For this review, take the finished solid that the model builds, in its own axes (mm). Face numbers are marked on the shaded views. A direction names the side the tool comes from. Round coordinates to 2 decimals unless told otherwise and drop trailing zeros. Order: outer loops, then holes, each group sorted by start corner. A loop starts at its lowest first (then second) coordinate and runs counter-clockwise, first axis right, second up. Notation, with made-up numbers: (8, -6) - (31, -6) arc R12 ccw to (31, 14) - close; hole circle Ø10 at (87, -4). An arc over 180 degrees is marked (long way). Write each question's results on one line, items separated by ' | '. Start each with the question number.
(1) Take a section at B-B, the plane z = -31.5. Give the number of separate pieces and of enclosed holes in the cut face, plus the area to 3 significant figures.
(2) Insertion check: pin 1 Ø4.5 at (x, z) = (35, -10) entering from +Y; pin 2 Ø6.5 at (x, z) = (35, -30) entering from +Y; pin 3 Ø4 at (x, z) = (8, -21) entering from -Y; pin 4 Ø10.5 at (x, z) = (37, -20.5) entering from -Y. Each pin has a flat end and moves straight along its axis. Give the tip position at first contact, or say it passes through.
(3) For the marked faces 5 and 6, list the 3-axis set-ups (+Z, -Z, +X, -X, +Y, -Y) from which the entire face can be reached by the end or side of a thin tool; tool diameter is ignored.
(4) For L1, parallel to Z at x = 35, y = 12; L2, parallel to X at y = 9.75, z = -30; L3, parallel to Z at x = 14.5, y = 7.75, list the stretches that pass through material, from the lowest coordinate up. Write a range as from..to.
(5) Draft analysis for pull direction Z (two halves, no side actions). For the marked faces 1, 2, 3 and 4, state which applies: pulls with the +Z half, pulls with the -Z half, needs draft (parallel to the pull), parting line crosses it, or undercut.
(6) Take a section at A-A, the plane x = 35. Give the boundary of the cut face in (y, z), plus the area to 3 significant figures.
```python
from build123d import *

# Parameters (mm, degrees)
BOSS_EXTRUDE1_DEPTH          = 40
F_5_0_5_DIAMETER_HOLE1_D     = 5
F_5_0_5_DIAMETER_HOLE1_DEPTH = 19
F_5_0_5_DIAMETER_HOLE1_TIP   = 1.502151548
FILLET1_R                    = 1
M6_CLEARANCE_HOLE3_D         = 6.6
M6_CLEARANCE_HOLE4_D         = 6.6
M6_CLEARANCE_HOLE4_DEPTH     = 19
M6_CLEARANCE_HOLE4_TIP       = 1.982840043
CUT_EXTRUDE2_START           = -10
SKETCH16_R                   = 7.2
CUT_EXTRUDE2_DEPTH           = 5.615550972
CUT_EXTRUDE3_START           = -10
SKETCH17_R                   = 7.2
CUT_EXTRUDE3_DEPTH           = 5.615550972


with BuildPart() as part:
    # Sketch1 → Boss-Extrude1 (new body)
    with BuildSketch(Plane.XY):
        Polygon((0, 0), (0, 15), (70, 15), (70, 0), (40, 6.926045734), (30, 6.926045734), align=None)
    extrude(amount=-BOSS_EXTRUDE1_DEPTH)

    # Ø5.0 (5) Diameter Hole1
    with Locations(Plane(origin=(0, 15, 0), x_dir=(1, 0, 0), z_dir=(0, 1, 0))):
        with Locations((35, 10), (35, 30)):
            Hole(F_5_0_5_DIAMETER_HOLE1_D / 2, depth=F_5_0_5_DIAMETER_HOLE1_DEPTH)
            with Locations((0, 0, -(F_5_0_5_DIAMETER_HOLE1_DEPTH + F_5_0_5_DIAMETER_HOLE1_TIP / 2))):  # 118° drill point
                Cone(0, F_5_0_5_DIAMETER_HOLE1_D / 2, F_5_0_5_DIAMETER_HOLE1_TIP, mode=Mode.SUBTRACT)

    # Fillet1
    fillet1_edges = [part.edges().sort_by_distance(p)[0] for p in [
        (55, 3.463022867, -40),
        (0, 0, -20),
        (70, 0, -20),
        (40, 6.926045734, -20),
        (30, 6.926045734, -20),
        (70, 7.5, -40),
        (0, 7.5, -40),
        (15, 3.463022867, -40),
        (0, 7.5, 0),
        (70, 7.5, 0),
        (35, 6.926045734, -40),
        (55, 3.463022867, 0),
        (35, 6.926045734, 0),
        (15, 3.463022867, 0),
    ]]
    fillet(fillet1_edges, radius=FILLET1_R)

    # M6 Clearance Hole3 (through all)
    with Locations(Plane(origin=(0, 0, 0), x_dir=(-0.974370065, -0.224951054, 0), z_dir=(0.224951054, -0.974370065, 0))):
        with Locations((-14.957172299, 10), (-14.957172299, 30)):
            Hole(M6_CLEARANCE_HOLE3_D / 2)

    # M6 Clearance Hole4
    with Locations(Plane(origin=(3.54220838, 15.342990138, 0), x_dir=(-0.974370065, 0.224951054, 0), z_dir=(-0.224951054, -0.974370065, 0))):
        with Locations((-53.248732236, 10), (-53.248732236, 30)):
            Hole(M6_CLEARANCE_HOLE4_D / 2, depth=M6_CLEARANCE_HOLE4_DEPTH)
            with Locations((0, 0, -(M6_CLEARANCE_HOLE4_DEPTH + M6_CLEARANCE_HOLE4_TIP / 2))):  # 118° drill point
                Cone(0, M6_CLEARANCE_HOLE4_D / 2, M6_CLEARANCE_HOLE4_TIP, mode=Mode.SUBTRACT)

    # Sketch16 → Cut-Extrude2 (cut, through all)
    with BuildSketch(Plane(origin=(0, 0, 0), x_dir=(0.974370065, 0.224951054, 0), z_dir=(0.224951054, -0.974370065, 0)).offset(CUT_EXTRUDE2_START)):
        with Locations((14.957172299, -10)):
            Circle(SKETCH16_R)
        with Locations((14.957172299, -30)):
            Circle(SKETCH16_R)
    extrude(amount=-CUT_EXTRUDE2_DEPTH, mode=Mode.SUBTRACT)

    # Sketch17 → Cut-Extrude3 (cut, through all)
    with BuildSketch(Plane(origin=(3.54220838, 15.342990138, 0), x_dir=(0.974370065, -0.224951054, 0), z_dir=(-0.224951054, -0.974370065, 0)).offset(CUT_EXTRUDE3_START)):
        with Locations((53.248732236, -10)):
            Circle(SKETCH17_R)
        with Locations((53.248732236, -30)):
            Circle(SKETCH17_R)
    extrude(amount=-CUT_EXTRUDE3_DEPTH, mode=Mode.SUBTRACT)


solid = part.part
```
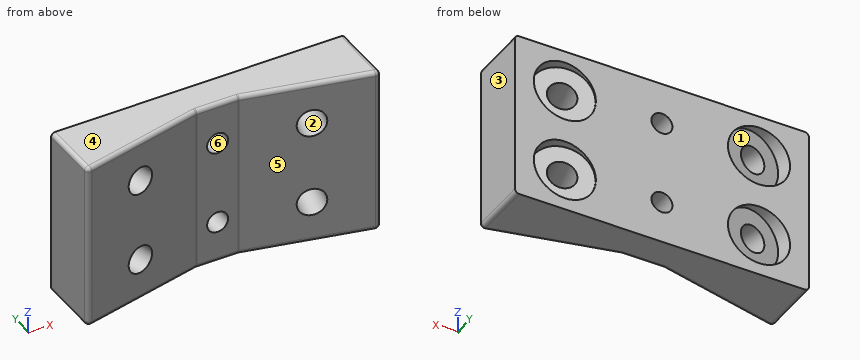
Results below:
1) separate pieces: 4 | enclosed holes: 0 | area: 568 mm^2
2) pin 1: passes through | pin 2: stops at y = 15 | pin 3: stops at y = 1.39 | pin 4: stops at y = 6.41
3) face 5: +Z, -Z, -Y | face 6: +Y, -Y
4) L1: z = -40..-32.5, -27.5..-12.5, -7.5..0 | L2: x = 0..9.71, 16.49..32.5, 37.5..53.51, 60.29..70 | L3: z = -40..-33.17, -26.83..-13.17, -6.83..0
5) face 1: undercut | face 2: undercut | face 3: needs draft | face 4: pulls with the +Z half
6) outline: (6.93, -39) arc R1 ccw to (7.93, -40) - (15, -40) - (15, -32.5) - (6.93, -32.5) - close; (6.93, -27.5) - (15, -27.5) - (15, -12.5) - (6.93, -12.5) - close; (6.93, -7.5) - (15, -7.5) - (15, 0) - (7.93, 0) arc R1 ccw to (6.93, -1) - close | area: 242 mm^2
